Could you check a few things on this model? Use its own coordinates, in mm. Face numbers are marked on the shaded views. A direction names the side the tool comes from. Round coordinates to 2 decimals unless told otherwise and drop trailing zeros. Loops run counter-clockwise (first coordinate to the right, second up) from the corner with the lowest first, then second, coordinate; pieces in that order, holes last.
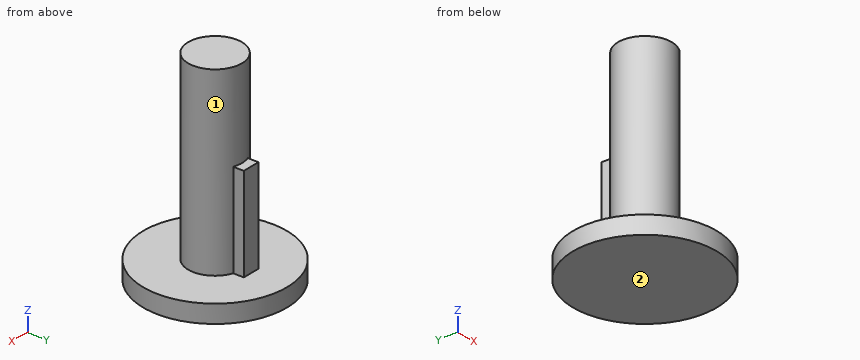
from build123d import *

# Parameters (mm, degrees)
SKETCH1_R           = 3
BOSS_EXTRUDE1_DEPTH = 20.29
SKETCH2_W           = 2
SKETCH2_H           = 1.17
BOSS_EXTRUDE2_DEPTH = 10.48
SKETCH3_R           = 8
BOSS_EXTRUDE3_DEPTH = 2


with BuildPart() as part:
    # Sketch1 → Boss-Extrude1 (new body)
    with BuildSketch(Plane.XY):
        Circle(SKETCH1_R)
    extrude(amount=BOSS_EXTRUDE1_DEPTH)

    # Sketch2 → Boss-Extrude2 (add)
    with BuildSketch(Plane(origin=(0, 0, 0), x_dir=(-1, 0, 0), z_dir=(0, 0, -1))):
        with Locations((0, 3.413427125)):
            Rectangle(SKETCH2_W, SKETCH2_H)
    extrude(amount=-BOSS_EXTRUDE2_DEPTH)

    # Sketch3 → Boss-Extrude3 (add)
    with BuildSketch(Plane(origin=(0, 0, 0), x_dir=(-1, 0, 0), z_dir=(0, 0, -1))):
        Circle(SKETCH3_R)
    extrude(amount=BOSS_EXTRUDE3_DEPTH)


solid = part.part
Item 1: Will these pins go through, and if not, where does the flat tip stop? pin 1 (3 mm diameter, centred on x = -5, y = -4, fed in from +Z); pin 2 (1.6 mm diameter, centred on x = -0.5, z = 5.5, fed in from +Y); pin 3 (6 mm diameter, centred on x = -2, z = 5, fed in from -Y).
Results list:
pin 1: stops at z = 0
pin 2: stops at y = 4
pin 3: stops at y = -3
Item 2: If we section it at A-A, the plane x = 0: Please give me the cut outline in (y, z), then the cut area to 3 significant figures.
Results list:
outline: (-8, -2) - (8, -2) - (8, 0) - (4, 0) - (4, 10.48) - (3, 10.48) - (3, 20.29) - (-3, 20.29) - (-3, 0) - (-8, 0) - close
area: 164 mm2
Item 3: If I drill on line 1 along Z through (x, y) = (-7, 3); line 2 along Y through (x, z) = (2.5, 12.25); line 3 along X through (y, z) = (-1.5, 15), over which ranges is the centre line in solid material (lowest first)?
Results list:
line 1: z = -2 to 0
line 2: y = -1.66 to 1.66
line 3: x = -2.6 to 2.6
Item 4: If we section it at D-D, the plane z = 18.25: Please give me the cut outline in (x, y).
Results list:
outline: circle Ø6 at (0, 0)
Item 5: If we section it at C-C, the plane z = 9: Please give me the cut outline in (x, y).
Results list:
outline: (-1, 2.83) arc R3 ccw (long way) to (1, 2.83) - (1, 4) - (-1, 4) - close
Item 6: If we section it at B-B, the plane y = 0: Please give me the cut outline in (x, z), then the cut area to 3 significant figures.
Results list:
outline: (-8, -2) - (8, -2) - (8, 0) - (3, 0) - (3, 20.29) - (-3, 20.29) - (-3, 0) - (-8, 0) - close
area: 154 mm2
Item 7: For the marked faces 1 and 2, which set-ups out of +Z, -Z, +X, -X, +Y, -Y let a thin tool reach every point of the face, with its end or its side?
Results list:
face 1: +Z
face 2: -Z, +X, -X, +Y, -Y
